Answer from the drawing. Dimensions are ordinates in mm from the lowest x, y and z of the part. Round coordinates to 2 decimals unless told otherwise and drop trailing zeros. Loops run counter-clockwise (first coordinate to the right, second up) from the corner with the lowest first, then second, coordinate; pieces in that order, holes last. Notation, with made-up numbers: (-37, 76) - (-2, 76) arc R25 ccw to (-2, 98) - close; hole circle Ø2 at (1, -9.75). An arc over 180 degrees is marked (long way). Write item = value, one per line. Start each with the question number.
1) Section D-D, the plane z = 251 is taken. Determine the outline of the cut face in (x, y) (3 decimals).
2) Given pin 1 Ø2 at (x, z) = (726, 137) entering from -Y (3 decimals), flat-ended and moving along its own axis, determine where the tip first touches the part or whether it passes through.
3) Section B-B, the plane y = 512 is taken. Determine the outline of the cut face in (x, z), and give its area (3 significant figures).
4) Section C-C, the plane x = 863.6 is taken. Determine the outline of the cut face in (y, z) (3 decimals), and give its area (3 significant figures).
5) Section A-A, the plane z = 558.8 is taken. Determine the outline of the cut face in (x, y) (3 decimals).
6) A straight line is drawn through the part: line 1 along Y through (x, z) = (328, 398) (3 decimals). Find the intervals that lie inside material, in ascending order.
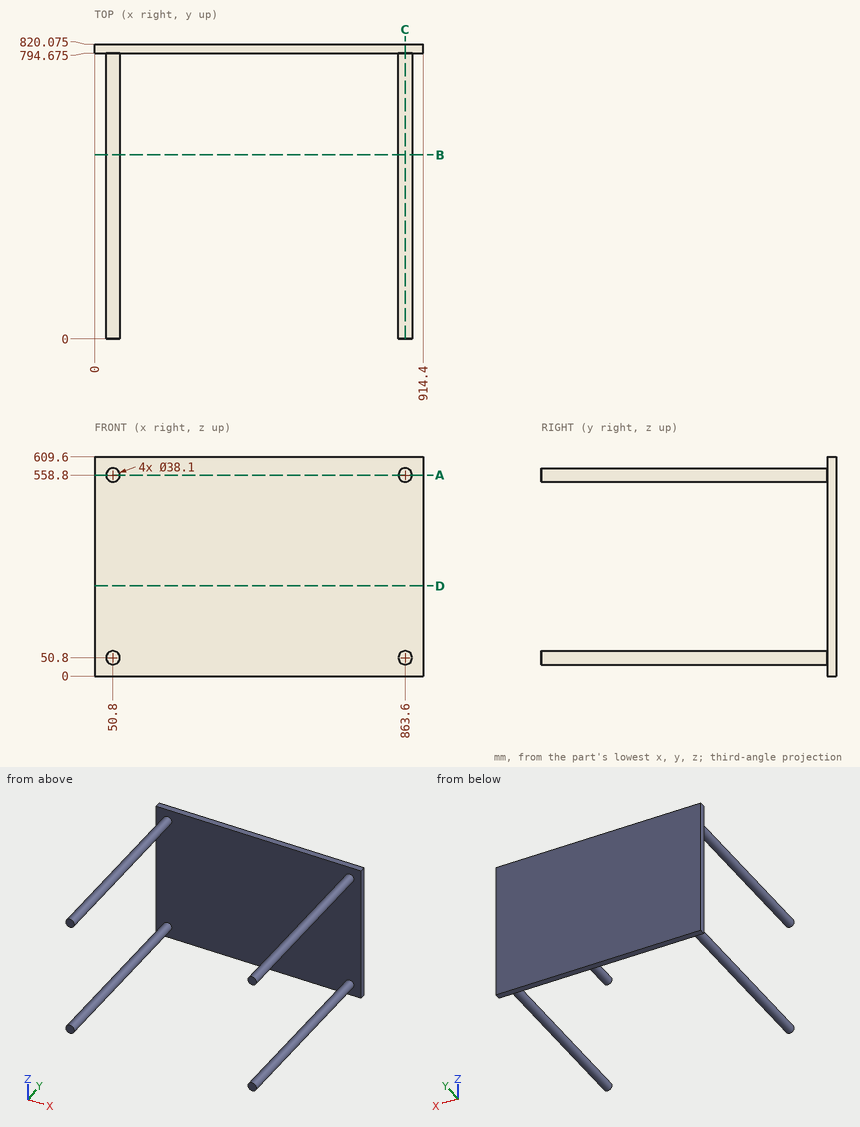
Geometry check:
q1.outline = (0, 794.675) - (914.4, 794.675) - (914.4, 820.075) - (0, 820.075) - close
q2.pin_1 = 794.675
q3.outline = circle Ø38.1 at (50.8, 50.8); circle Ø38.1 at (50.8, 558.8); circle Ø38.1 at (863.6, 50.8); circle Ø38.1 at (863.6, 558.8)
q3.area = 4,560 mm2
q4.outline = (0, 31.75) - (794.675, 31.75) - (794.675, 0) - (820.075, 0) - (820.075, 609.6) - (794.675, 609.6) - (794.675, 577.85) - (0, 577.85) - (0, 539.75) - (794.675, 539.75) - (794.675, 69.85) - (0, 69.85) - close
q4.area = 76,000 mm2
q5.outline = (0, 794.675) - (31.75, 794.675) - (31.75, 0) - (69.85, 0) - (69.85, 794.675) - (844.55, 794.675) - (844.55, 0) - (882.65, 0) - (882.65, 794.675) - (914.4, 794.675) - (914.4, 820.075) - (0, 820.075) - close
q6.line_1 = 794.675 to 820.075
